The drawing under review shows one solid part. Ordinate dimensions are in mm from its lowest x, y, z. Give positions to 0.01 mm unless a question says otherwise; leave off trailing zeros. One line per item, written item: value. Start each with the question number.
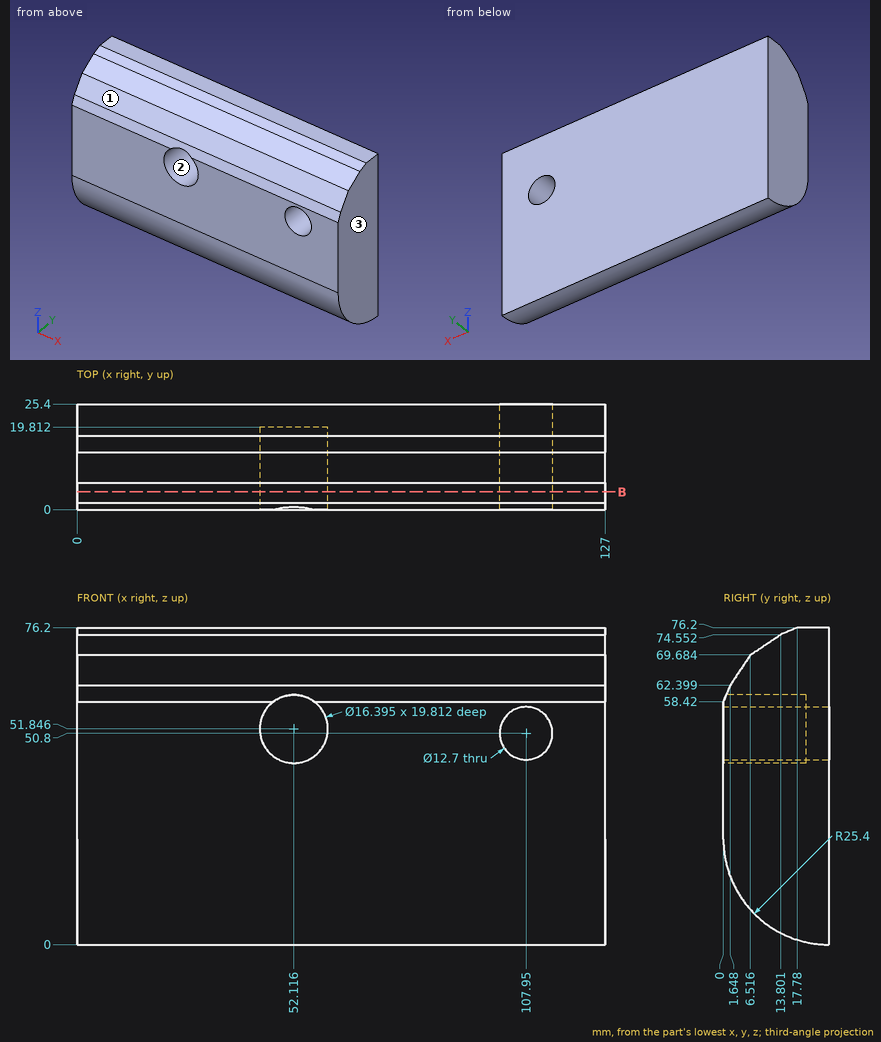
Q1. Wall thickness on line 1 (X direction, y = 6, z = 51.5) (1 decimal); line 2 (Y direction, x = 51, z = 48.5); line 3 (Z direction, x = 110, y = 3) (1 decimal): over which ranges is each line inside the solid? List them lowest first. Write a range as from..to.
Q2. For P1, Ø5, axis at x = 50.5, z = 54, coming from the -Y side; P2, Ø5, axis at x = 81, y = 13, coming from the +Z side (1 decimal); P3, Ø3, axis at x = 94, z = 17.5, coming from the -Y side, all flat-tipped, find the tip position at first contact; note any pin that passes through.
Q3. The part is to be moulded in two halves that separate along X. For the marked faces 1, 2 and 3, say which applies: pulls with the +X half, pulls with the -X half, needs draft (parallel to the pull), parting line crosses it, or undercut.
Q4. Take a section at B-B, the plane y = 4.25. State how many separate pieces and enclosed holes the cut face has, then the cut area to 3 significant figures.
Results list:
1. line 1: x = 0..43.9, 60.3..101.6, 114.3..127
1. line 2: y = 19.81..25.4
1. line 3: z = 13.4..44.8, 56.8..64.4
2. P1: stops at y = 19.81
2. P2: stops at z = 75.3
2. P3: stops at y = 0.82
3. face 1: needs draft
3. face 2: undercut
3. face 3: pulls with the +X half
4. separate pieces: 1
4. enclosed holes: 2
4. area: 6,640 mm^2
